Input: part model. Units: mm. Frame: model coordinates. A direction names the side the tool comes from. Coordinates: 2 decimals unless noted, no trailing zeros. Order: outer loops, then holes, each group sorted by start corner. A loop starts at its lowest first (then second) coordinate and runs counter-clockwise, first axis right, second up.
from build123d import *

# Parameters (mm, degrees)
F1_DEPTH = 10


with BuildPart() as f1:
    # F0 (on Front) → F1 (new body)
    with BuildSketch(Plane.XZ):
        with BuildLine():
            Line((6.51253, 105.134805), (0, 105.134805))
            Line((0, 105.134805), (-10.789488, 105.134805))
            ThreePointArc((-10.789488, 105.134805), (-14.298656, 104.077086), (-16.63878, 101.256299))
            Line((-16.63878, 101.256299), (-32.478897, 63.767443))
            Line((-32.478897, 63.767443), (-38.307014, 63.767443))
            ThreePointArc((-38.307014, 63.767443), (-42.797142, 61.907571), (-44.657014, 57.417443))
            Line((-44.657014, 57.417443), (-44.657014, 0))
            Line((-44.657014, 0), (-42.657014, 0))
            Line((-42.657014, 0), (-42.657014, -12.672931))
            Line((-42.657014, -12.672931), (-44.657014, -12.672931))
            Line((-44.657014, -12.672931), (-44.657014, -54.299037))
            ThreePointArc((-44.657014, -54.299037), (-42.797142, -58.789165), (-38.307014, -60.649037))
            Line((-38.307014, -60.649037), (0, -60.649037))
            Line((0, -60.649037), (36.564393, -60.649037))
            ThreePointArc((36.564393, -60.649037), (41.054521, -58.789165), (42.914393, -54.299037))
            Line((42.914393, -54.299037), (42.914393, -12.672931))
            Line((42.914393, -12.672931), (40.914393, -12.672931))
            Line((40.914393, -12.672931), (40.914393, 0))
            Line((40.914393, 0), (42.914393, 0))
            Line((42.914393, 0), (42.914393, 58.767443))
            ThreePointArc((42.914393, 58.767443), (41.449927, 62.302977), (37.914393, 63.767443))
            Line((37.914393, 63.767443), (32.005376, 63.767443))
            Line((32.005376, 63.767443), (10.90388, 102.52563))
            ThreePointArc((10.90388, 102.52563), (9.066535, 104.4333), (6.51253, 105.134805))
        make_face()
    extrude(amount=F1_DEPTH)


solid = f1.part
Item 1: Cut plane B-B on z = -5. Return loops of the section in (x, y).
Response values:
outline: (-42.66, -10) - (40.91, -10) - (40.91, 0) - (-42.66, 0) - close
Item 2: Access query for faces 1 (the face through (-44.657, -5, -33)), 2 (the face through (-42.657, -5, -6)), 3 (the face through (-35, -5, 63.767)), 4 (the face through (35, -5, 63.767)), 5 (the face through (-2, -5, 105.135)). Directions: +Z, -Z, +X, -X, +Y, -Y. A direction counts if a zero-diameter tool reaches every point of the face in a straight line with its end or side. Return the directions, or none.
Response values:
face 1: +Z, -Z, -X, +Y, -Y
face 2: -X, +Y, -Y
face 3: +Z, -X, +Y, -Y
face 4: +Z, +X, +Y, -Y
face 5: +Z, +X, -X, +Y, -Y
Item 3: Pin query (flat end, axial travel): pin 1 Ø1 at (x, y) = (41.5, -6.5) entering from -Z; pin 2 Ø1.8 at (x, y) = (34, -5) entering from +Z; pin 3 Ø1.5 at (y, z) = (-4, 62.5) entering from +X; pin 4 Ø1.5 at (x, z) = (-35.5, 32.5) entering from +Y. Return the tip coordinate at first contact, or that it passes through.
Response values:
pin 1: stops at z = -58.84
pin 2: stops at z = 63.77
pin 3: stops at x = 41.93
pin 4: stops at y = 0
Item 4: Ray query, probe 1 along Z at (x, y) = (32, -7.25); probe 2 along Z at (x, y) = (-15.5, -7.75); probe 3 along X at (y, z) = (-9.5, 94.5). Return the intervals inside material, ascending.
Response values:
probe 1: z = -60.65 to 63.78
probe 2: z = -60.65 to 103.04
probe 3: x = -19.49 to 15.27
Item 5: Draft query along Z for faces 6 (the face through (40.914, -5, -6)), 7 (the face through (42.914, -5, 29)), 8 (the face through (-14.255, -4.93, 104.106)). Return one class per face: pulls with the +Z half, pulls with the -Z half, needs draft (parallel to the pull), parting line crosses it, or undercut.
Response values:
face 6: undercut
face 7: needs draft
face 8: pulls with the +Z half
Item 6: Cut plane A-A on y = -7. Return loops of the section in (x, z), then the cut area to 3 significant figures.
Response values:
outline: (-44.66, -54.3) arc R6.35 ccw to (-38.31, -60.65) - (36.56, -60.65) arc R6.35 ccw to (42.91, -54.3) - (42.91, -12.67) - (40.91, -12.67) - (40.91, 0) - (42.91, 0) - (42.91, 58.77) arc R5 ccw to (37.91, 63.77) - (32.01, 63.77) - (10.9, 102.53) arc R5 ccw to (6.51, 105.13) - (-10.79, 105.13) arc R6.35 ccw to (-16.64, 101.26) - (-32.48, 63.77) - (-38.31, 63.77) arc R6.35 ccw to (-44.66, 57.42) - (-44.66, 0) - (-42.66, 0) - (-42.66, -12.67) - (-44.66, -12.67) - close
area: 12,600 mm2
Item 7: Cut plane C-C on x = -24.5. Return loops of the section in (y, z).
Response values:
outline: (-10, -60.65) - (0, -60.65) - (0, 82.65) - (-10, 82.65) - close
